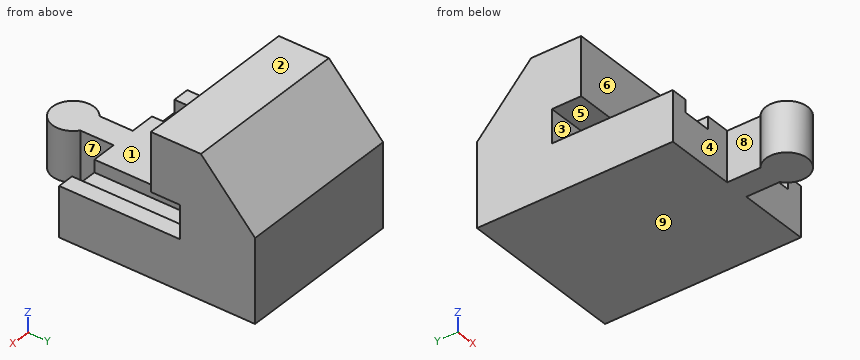
```python
from build123d import *

# Parameters (mm, degrees)
PAD_DEPTH    = 20
PAD001_DEPTH = 6


with BuildPart() as part:
    # AdditivePipe: sweep along a path in Sketch
    with BuildLine(Plane.XY) as additivepipe_path:
        Line((0, 0), (0, 47))
    # Sketch001 → AdditivePipe (sweep)
    with BuildSketch(Plane.XZ):
        Polygon((-20, 6), (-20, -6), (-16, -6), (-9, -6), (9, -6), (16, -6), (20, -6), (20, 6), (16, 6), (16, 3), (9, 3), (9, 6), (-9, 6), (-9, 3), (-16, 3), (-16, 6), align=None)
    sweep(path=additivepipe_path.line)

    # Sketch002 → Pad (new body, symmetric)
    with BuildSketch(Plane.YZ):
        Polygon((47, 3), (47, 14), (34, 28), (22, 28), (22, 14), (29, 14), (29, 3), align=None)
    extrude(amount=PAD_DEPTH, both=True)

    # Sketch003 → Pad001 (join, symmetric)
    with BuildSketch(Plane.XY):
        with BuildLine():
            Line((-3, 0), (3, 0))
            Line((3, 0), (3, -8))
            ThreePointArc((-3, -8), (0, -17), (3, -8))
            Line((-3, 0), (-3, -8))
        make_face()
    extrude(amount=PAD001_DEPTH, both=True)


solid = part.part
```
Could you check a few things on this model? Use its own coordinates, in mm. Face numbers are marked on the shaded views. A direction names the side the tool comes from. Coordinates: 2 decimals unless noted, no trailing zeros. Loops run counter-clockwise (first coordinate to the right, second up) from the corner with the lowest first, then second, coordinate; pieces in that order, holes last. Notation, with made-up numbers: M 2.25,24.25 L 13.25,24.25 A20 cw 13.25,39.25 Z; hole C 36,84.5 d4. An arc over 180 degrees is marked long. Put each result on its own line as item: value. Start each with the question number.
(1) Will these pins go through, and if not, where does the flat tip stop? P1, Ø4, axis at y = 20.5, z = 14.5, coming from the -X side; P2, Ø2.5, axis at y = -3, z = -1, coming from the +X side; P3, Ø2, axis at x = -3, z = 6.5, coming from the -Y side; P4, Ø15.5, axis at x = -7.5, z = 19.5, coming from the -Y side.
(2) Suppose I cut it at C-C on y = 9.5. Please give me the cut outline in (x, z), then the cut area to 3 significant figures.
(3) Thinking about a two-plate mould opening in Z: for the marked faces 1, 2, 3 and 4, which applies, pulls with the +Z half, pulls with the -Z half, needs draft (parallel to the pull), parting line crosses it, or undercut?
(4) For the marked faces 5, 6, 7, 8 and 9, which set-ups out of +Z, -Z, +X, -X, +Y, -Y let a thin tool reach every point of the face, with its end or its side?
(5) Suppose I cut it at B-B on z = 0.5. Please give me the cut outline in (x, y).
(6) I need wall thicknesses on line 1 (X direction, y = 7, z = 5); line 2 (Z direction, x = 0, y = 27); line 3 (Y direction, x = -14.5, z = -1.5). Which ranges of each line are inside material? Lowest first, please. Write a range as from..to.
(7) Suppose I cut it at A-A on y = 26. Please give me the cut outline in (x, z).
(8) Suppose I cut it at D-D on x = 10. Please give me the cut outline in (y, z).
Solutions:
1. P1: stops at x = -20
1. P2: stops at x = 3
1. P3: stops at y = -16.52
1. P4: stops at y = 22
2. outline: M -20,-6 L 20,-6 L 20,6 L 16,6 L 16,3 L 9,3 L 9,6 L -9,6 L -9,3 L -16,3 L -16,6 L -20,6 Z
2. area: 438 mm2
3. face 1: undercut
3. face 2: pulls with the +Z half
3. face 3: undercut
3. face 4: needs draft
4. face 5: +X, -X, -Y
4. face 6: +Z, +X, -X, -Y
4. face 7: +Z, -Z, +X
4. face 8: +Z, -Z, -X
4. face 9: -Z, +X, -X, +Y, -Y
5. outline: M -20,0 L -3,0 L -3,-8 A5 ccw long 3,-8 L 3,0 L 20,0 L 20,47 L -20,47 Z
6. line 1: x = -20..-16, -9..9, 16..20
6. line 2: z = -6..6, 14..28
6. line 3: y = 0..47
7. outline: M -20,-6 L 20,-6 L 20,6 L 16,6 L 16,3 L 9,3 L 9,6 L -9,6 L -9,3 L -16,3 L -16,6 L -20,6 Z; M -20,14 L 20,14 L 20,28 L -20,28 Z
8. outline: M 0,-6 L 47,-6 L 47,14 L 34,28 L 22,28 L 22,14 L 29,14 L 29,3 L 0,3 Z
